Check sheet for the drawn part. Datum: minimum x, y, z corner. Units: mm. Give positions to 0.01 mm unless a question says otherwise; leave off trailing zeros. Write each loop counter-clockwise with the first axis right and the second up, starting at its lowest first coordinate (ties: lowest second). Pieces come first, ordered by that corner, then holes. Notation, with made-up numbers: M 22,-15 L 52,-15 A20 ccw 52,-4 Z; hole C 61.5,67.5 d10. An arc over 180 degrees is marked long. Write item = value, one per line. Start each with the question number.
1) Gauge pin test, flat end, axial feed: pin 1 (8 mm diameter, centred on x = 31.5, z = 49.5, fed in from -Y). Record the tip position at first contact, or that the pin passes through.
2) Sectioned sample at A-A, the plane z = 16.5. Record the cut outline in (x, y), then the cut area to 3 significant figures.
3) Sectioned sample at D-D, the plane z = 49.5. Record the cut outline in (x, y), then the cut area to 3 significant figures.
4) Sectioned sample at C-C, the plane y = 2. Count the separate pieces of the cut face and the enclosed holes in it, then the cut area to 3 significant figures.
5) Sectioned sample at B-B, the plane x = 13.5. Record the cut outline in (y, z).
6) Scan lines: L1, parallel to Z at x = 13.5, y = 3.25; L2, parallel to X at y = 5.25, z = 49.5; L3, parallel to Z at x = 68.5, y = 5.4. Record each from-to range of solid material in increasing order.
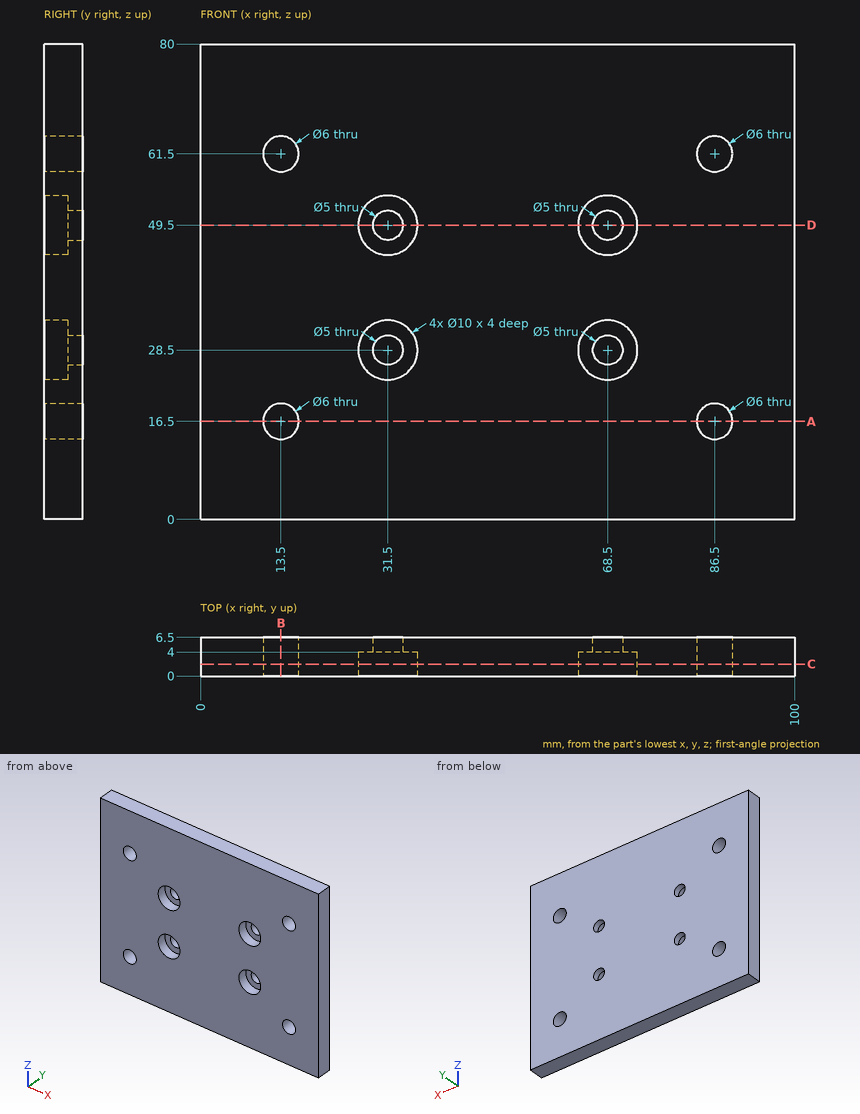
Data:
q1.pin_1 = 4
q2.outline = M 0,0 L 10.5,0 L 10.5,6.5 L 0,6.5 Z; M 16.5,0 L 83.5,0 L 83.5,6.5 L 16.5,6.5 Z; M 89.5,0 L 100,0 L 100,6.5 L 89.5,6.5 Z
q2.area = 572 mm2
q3.outline = M 0,0 L 26.5,0 L 26.5,4 L 29,4 L 29,6.5 L 0,6.5 Z; M 34,4 L 36.5,4 L 36.5,0 L 63.5,0 L 63.5,4 L 66,4 L 66,6.5 L 34,6.5 Z; M 71,4 L 73.5,4 L 73.5,0 L 100,0 L 100,6.5 L 71,6.5 Z
q3.area = 545 mm2
q4.separate_pieces = 1
q4.enclosed_holes = 8
q4.area = 7,570 mm2
q5.outline = M 0,0 L 6.5,0 L 6.5,13.5 L 0,13.5 Z; M 0,19.5 L 6.5,19.5 L 6.5,58.5 L 0,58.5 Z; M 0,64.5 L 6.5,64.5 L 6.5,80 L 0,80 Z
q6.L1 = 0 to 13.5, 19.5 to 58.5, 64.5 to 80
q6.L2 = 0 to 29, 34 to 66, 71 to 100
q6.L3 = 0 to 26, 31 to 47, 52 to 80
